The listing builds one solid part. Answer for the finished solid, in the listing's coordinates (mm). Face numbers are marked on the shaded views. A direction names the side the tool comes from. Coordinates: 2 decimals unless noted, no trailing zeros. Write each loop counter-clockwise with the first axis right and the second up, starting at its lowest first coordinate (ties: lowest second). Pieces come first, ordered by that corner, then holes.
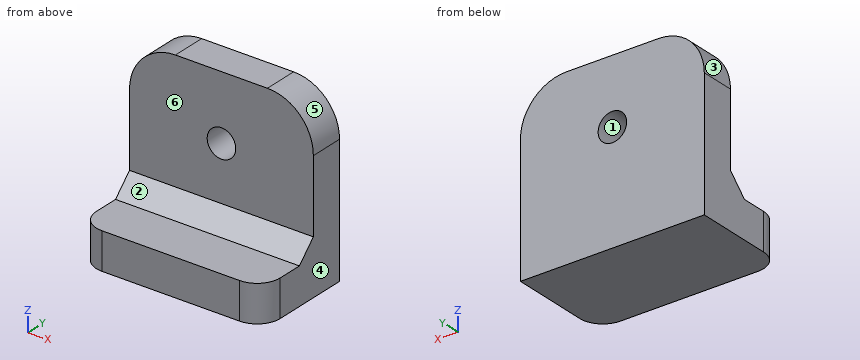
from build123d import *

# Parameters (mm, degrees)
SKETCH1_W           = 40
SKETCH1_H           = 22
BOSS_EXTRUDE1_DEPTH = 8
SKETCH2_W           = 40
SKETCH2_H           = 7.5
BOSS_EXTRUDE2_DEPTH = 30
CHAMFER1_SIZE       = 4
FILLET1_R           = 10
FILLET2_R           = 5
SKETCH3_R           = 3.1
CUT_EXTRUDE1_DEPTH  = 49.249352327


with BuildPart() as part:
    # Sketch1 → Boss-Extrude1 (new body)
    with BuildSketch(Plane.XY):
        with Locations((0, -15.406470283)):
            Rectangle(SKETCH1_W, SKETCH1_H)
    extrude(amount=BOSS_EXTRUDE1_DEPTH)

    # Sketch2 → Boss-Extrude2 (add)
    with BuildSketch(Plane.XY.offset(8)):
        with Locations((0, -8.156470283)):
            Rectangle(SKETCH2_W, SKETCH2_H)
    extrude(amount=BOSS_EXTRUDE2_DEPTH)

    # Chamfer1
    chamfer1_edges = [part.edges().sort_by_distance(p)[0] for p in [
        (0, -11.906470283, 8),
    ]]
    chamfer(chamfer1_edges, length=CHAMFER1_SIZE)

    # Fillet1
    fillet1_edges = [part.edges().sort_by_distance(p)[0] for p in [
        (-20, -8.156470283, 38),
        (20, -8.156470283, 38),
    ]]
    fillet(fillet1_edges, radius=FILLET1_R)

    # Fillet2
    fillet2_edges = [part.edges().sort_by_distance(p)[0] for p in [
        (20, -26.406470283, 4),
        (-20, -26.406470283, 4),
    ]]
    fillet(fillet2_edges, radius=FILLET2_R)

    # Sketch3 → Cut-Extrude1 (cut, through all)
    with BuildSketch(Plane(origin=(0, -4.406470283, 0), x_dir=(1, 0, 0), z_dir=(0, 1, 0))):
        with Locations(Location((0, -23.851791769, 0), (0, 0, 270))):
            Circle(SKETCH3_R)
    extrude(amount=-CUT_EXTRUDE1_DEPTH, mode=Mode.SUBTRACT)


solid = part.part
1. For a pull along X with two mould halves and no side action, classify the marked faces 1, 2, 3 and 4 as pulls with the +X half, pulls with the -X half, needs draft (parallel to the pull), parting line crosses it, or undercut.
Results found:
face 1: undercut
face 2: needs draft
face 3: pulls with the -X half
face 4: pulls with the +X half
2. Section B-B on z = 21.5 is taken. Give the vertices of the cut face in (x, y), then the cut area to 3 significant figures.
Results found:
outline: (-20, -11.91) - (-2.02, -11.91) - (-2.02, -4.41) - (-20, -4.41) - close; (2.02, -11.91) - (20, -11.91) - (20, -4.41) - (2.02, -4.41) - close
area: 270 mm2
3. Flat-ended cylindrical pins translate along their axes: P1, Ø5, axis at x = 2, y = -20, coming from the +Z side; P2, Ø4, axis at x = -15.5, z = 19.5, coming from the -Y side; P3, Ø3.5, axis at x = 0, z = 23.85, coming from the +Y side. Find the tip coordinate at first contact, or state that the pin passes through.
Results found:
P1: stops at z = 8
P2: stops at y = -11.91
P3: passes through
4. Section A-A on x = 0 is taken. Give the vertices of the cut face in (y, z), then the cut area to 4 significant figures.
Results found:
outline: (-26.41, 0) - (-4.41, 0) - (-4.41, 20.75) - (-11.91, 20.75) - (-11.91, 12) - (-15.91, 8) - (-26.41, 8) - close; (-11.91, 26.95) - (-4.41, 26.95) - (-4.41, 38) - (-11.91, 38) - close
area: 362.5 mm2
5. Section C-C on x = 6 is taken. Give the vertices of the cut face in (y, z).
Results found:
outline: (-26.41, 0) - (-4.41, 0) - (-4.41, 38) - (-11.91, 38) - (-11.91, 12) - (-15.91, 8) - (-26.41, 8) - close
6. Find the intervals of material crossed by L1, parallel to Z at x = 3, y = -19; L2, parallel to Y at x = 13.5, z = 13; L3, parallel to Z at x = 13, y = -14.25, in increasing order.
Results found:
L1: z = 0 to 8
L2: y = -11.91 to -4.41
L3: z = 0 to 9.66
7. Section D-D on z = 17 is taken. Give the vertices of the cut face in (x, y), then the cut area to 3 significant figures.
Results found:
outline: (-20, -11.91) - (20, -11.91) - (20, -4.41) - (-20, -4.41) - close
area: 300 mm2
8. A tool of negligible diameter and unlimited length cuts with its end or side. For the marked faces 5 and 6, from which of +Z, -Z, +X, -X, +Y, -Y can it reach the whole face along a straight path? Write none if from no direction.
Results found:
face 5: +Z, +X, +Y, -Y
face 6: +Z, +X, -X, -Y
